Answer from the drawing. Dimensions are ordinates in mm from the lowest x, y and z of the part. Round coordinates to 2 decimals unless told otherwise and drop trailing zeros. Write each loop counter-clockwise with the first axis right and the second up, starting at its lowest first coordinate (ties: lowest second). Pieces come first, ordered by that corner, then holes. Notation, with made-up numbers: (25.5, -18.75) - (62.5, -18.75) arc R34 cw to (62.5, 13.25) - close; hole circle Ø11 at (-21, 51). An arc over 180 degrees is marked (long way). Write item = value, one per line. Start each with the question number.
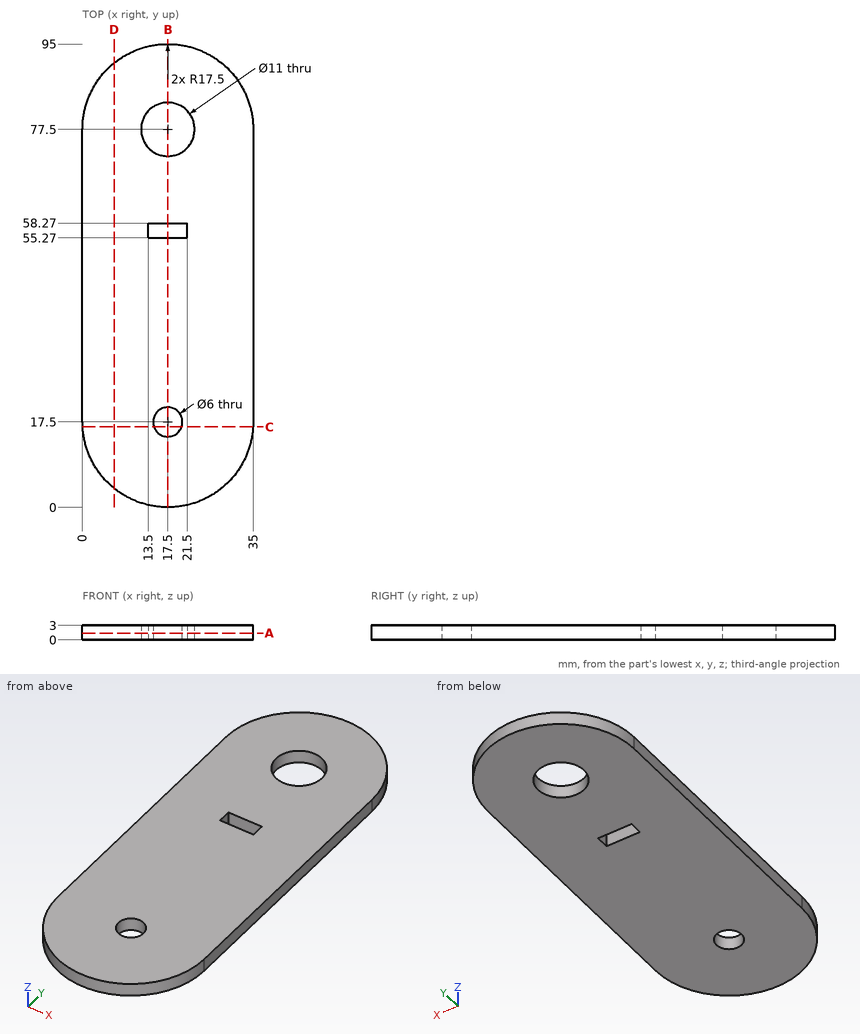
1. Consider line 1 (Y direction, x = 17.5, z = 1.8); line 2 (Y direction, x = 20, z = 1.8); line 3 (Y direction, x = 14, z = 2.4). Determine where each line is inside the solid, lowest interval first.
2. Find section B-B on x = 17.5. Give the vertices of the cut face in (y, z).
3. Find section A-A on z = 1.4. Give the vertices of the cut face in (x, y), plus the area to 3 significant figures.
4. Find section C-C on y = 16.5. Give the vertices of the cut face in (x, z).
5. Each of these flat-tipped pins is pushed along its axis until it touches: pin 1 (9.5 mm diameter, centred on x = 17.5, y = 17.5, fed in from +Z); pin 2 (1.5 mm diameter, centred on x = 19, z = 1.5, fed in from -Y). Where does it stop, or does it pass through?
6. Find section D-D on x = 6.5. Give the vertices of the cut face in (y, z), plus the area to 3 significant figures.
Answer key:
q1.line_1 = 0 to 14.5, 20.5 to 55.27, 58.27 to 72, 83 to 95
q1.line_2 = 0.18 to 15.84, 19.16 to 55.27, 58.27 to 72.6, 82.4 to 94.82
q1.line_3 = 0.35 to 55.27, 58.27 to 73.26, 81.74 to 94.65
q2.outline = (0, 0) - (14.5, 0) - (14.5, 3) - (0, 3) - close; (20.5, 0) - (55.27, 0) - (55.27, 3) - (20.5, 3) - close; (58.27, 0) - (72, 0) - (72, 3) - (58.27, 3) - close; (83, 0) - (95, 0) - (95, 3) - (83, 3) - close
q3.outline = (0, 17.5) arc R17.5 ccw to (35, 17.5) - (35, 77.5) arc R17.5 ccw to (0, 77.5) - close; hole circle Ø11 at (17.5, 77.5); hole (13.5, 55.27) - (21.5, 55.27) - (21.5, 58.27) - (13.5, 58.27) - close; hole circle Ø6 at (17.5, 17.5)
q3.area = 2,910 mm²
q4.outline = (0.03, 0) - (14.67, 0) - (14.67, 3) - (0.03, 3) - close; (20.33, 0) - (34.97, 0) - (34.97, 3) - (20.33, 3) - close
q5.pin_1 = 3
q5.pin_2 = 0.02
q6.outline = (3.89, 0) - (91.11, 0) - (91.11, 3) - (3.89, 3) - close
q6.area = 262 mm²
